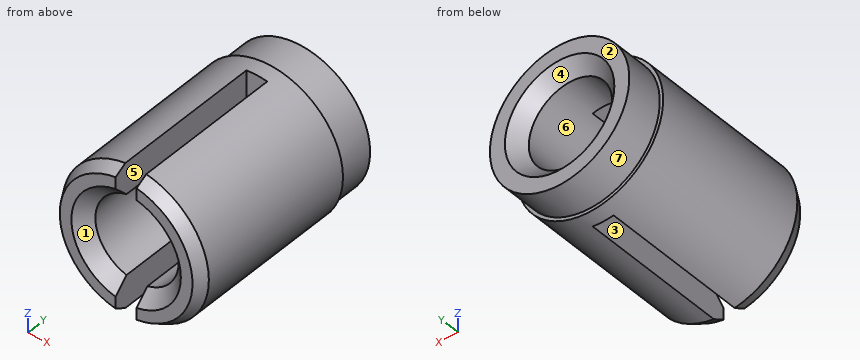
from build123d import *

# Parameters (mm, degrees)
SKETCH1_R           = 3.175
EXTRUDE1_DEPTH      = 9.525
EXTRUDE2_START      = -9.525
SKETCH1_4_R         = 3.3274
SKETCH1_4_R_2       = 3.175
EXTRUDE2_DEPTH      = 7.858125
EXTRUDE3_START      = -9.525
SKETCH4_R           = 1.897444252
EXTRUDE3_DEPTH      = 9.525
CHAMFER1_SIZE       = 0.5953125
CHAMFER2_SIZE       = 0.3048
CHAMFER2_SIZE2      = 0.527929086
SKETCH8_W           = 0.9525
SKETCH8_H           = 7.14375
EXTRUDE4_DEPTH      = 4.3274
EXTRUDE4_DEPTH_BACK = 4.3274


with BuildPart() as part:
    # Sketch1 → Extrude1 (new body)
    with BuildSketch(Plane(origin=(0, 0, 0), x_dir=(1, 0, 0), z_dir=(0, 1, 0))):
        Circle(SKETCH1_R)
    extrude(amount=-EXTRUDE1_DEPTH)

    # Sketch1<4> → Extrude2 (add)
    with BuildSketch(Plane(origin=(0, 0, 0), x_dir=(1, 0, 0), z_dir=(0, 1, 0)).offset(EXTRUDE2_START)):
        Circle(SKETCH1_4_R)
        Circle(SKETCH1_4_R_2, mode=Mode.SUBTRACT)
    extrude(amount=EXTRUDE2_DEPTH)

    # Sketch4 → Extrude3 (cut)
    with BuildSketch(Plane(origin=(0, 0, 0), x_dir=(1, 0, 0), z_dir=(0, 1, 0)).offset(EXTRUDE3_START)):
        Circle(SKETCH4_R)
    extrude(amount=EXTRUDE3_DEPTH, mode=Mode.SUBTRACT)

    # Chamfer1
    chamfer1_edges = [part.edges().sort_by_distance(p)[0] for p in [
        (-1.897444252, -9.525, 0),
        (-1.897444252, 0, 0),
    ]]
    chamfer(chamfer1_edges, length=CHAMFER1_SIZE)

    # Chamfer2
    chamfer2_edges = [part.edges().sort_by_distance(p)[0] for p in [
        (-3.3274, -9.525, 0),
    ]]
    chamfer2_side = [part.faces().sort_by_distance(p)[0] for p in [
        (-2.586869836, -9.525, 0),
    ]]
    chamfer(chamfer2_edges, length=CHAMFER2_SIZE, length2=CHAMFER2_SIZE2, reference=chamfer2_side[0])

    # Sketch8 → Extrude4 (cut, two sides)
    with BuildSketch(Plane.XY) as extrude4_sk:
        with Locations((0, -5.953125)):
            Rectangle(SKETCH8_W, SKETCH8_H)
    extrude(amount=EXTRUDE4_DEPTH, mode=Mode.SUBTRACT)
    extrude(extrude4_sk.sketch, amount=-EXTRUDE4_DEPTH_BACK, mode=Mode.SUBTRACT)


solid = part.part
Verification items for the finished model (mm, model axes). Face numbers are marked on the shaded views. A direction names the side the tool comes from. Coordinates: 2 decimals unless noted, no trailing zeros. Order: outer loops, then holes, each group sorted by start corner. A loop starts at its lowest first (then second) coordinate and runs counter-clockwise, first axis right, second up. Notation, with made-up numbers: (74.5, 63.5) -> (118.5, 63.5) arc R11 cw to (118.5, 79.5) -> close; hole circle Ø6 at (-17, 81). An arc over 180 degrees is marked (long way). Put each result on its own line as item: value. Start each with the question number.
1. Cross-section at B-B, the plane z = 0. Record the boundary of the cut face in (x, y) (3 decimals), then the cut area to 3 significant figures.
2. Access from +Z, -Z, +X, -X, +Y, -Y to the whole of each face (thin tool, end or side, straight path). Record for the marked faces 1, 2 and 3.
3. Mould release check, pull along Z, two halves, no side actions. Record for the marked faces 4, 5, 6 and 7: released by +Z, released by -Z, zero draft, split by the parting line, or undercut.
4. Cross-section at C-C, the plane x = 0. Record the boundary of the cut face in (y, z) (3 decimals).
5. Go/stop test with flat-tipped pins: pin 1 Ø0.7 at (y, z) = (-4.5, 2.5) entering from -X; pin 2 Ø3.5 at (x, z) = (0, 0) entering from +Y; pin 3 Ø1.5 at (y, z) = (-7, 1.5) entering from +X; pin 4 Ø0.8 at (x, z) = (0, -2.5) entering from -Y. Record where each tip stops, or that it passes through.
6. Material ranges on L1, parallel to X at y = -4.25, z = 0; L2, parallel to X at y = -8.75, z = -2.5, recorded low to high. Write a range as [from, to].
Computed:
1. outline: (-3.327, -8.997) -> (-3.023, -9.525) -> (-2.493, -9.525) -> (-1.897, -8.93) -> (-1.897, -0.595) -> (-2.493, 0) -> (-3.175, 0) -> (-3.175, -1.667) -> (-3.327, -1.667) -> close; (1.897, -8.93) -> (2.493, -9.525) -> (3.023, -9.525) -> (3.327, -8.997) -> (3.327, -1.667) -> (3.175, -1.667) -> (3.175, 0) -> (2.493, 0) -> (1.897, -0.595) -> close
1. area: 25.9 mm2
2. face 1: -Y
2. face 2: +Z, -Z, +X, -X, +Y
2. face 3: +Z, -Z, -Y
3. face 4: undercut
3. face 5: zero draft
3. face 6: undercut
3. face 7: split by the parting line
4. outline: (-2.381, -3.327) -> (-1.667, -3.327) -> (-1.667, -3.175) -> (0, -3.175) -> (0, -2.493) -> (-0.595, -1.897) -> (-2.381, -1.897) -> close; (-2.381, 1.897) -> (-0.595, 1.897) -> (0, 2.493) -> (0, 3.175) -> (-1.667, 3.175) -> (-1.667, 3.327) -> (-2.381, 3.327) -> close
5. pin 1: x = -2.54
5. pin 2: through
5. pin 3: x = 3.24
5. pin 4: y = -2.38
6. L1: [-3.33, -1.9], [1.9, 3.33]
6. L2: [-2.2, -0.48], [0.48, 2.2]
